The listing builds one solid part. Answer for the finished solid, in the listing's coordinates (mm). A direction names the side the tool comes from. Coordinates: 2 decimals unless noted, no trailing zeros. Order: outer loops, then holes, each group sorted by start corner. A loop starts at its lowest first (then second) coordinate and runs counter-clockwise, first axis right, second up. Notation, with made-up numbers: (65, 21.25) -> (120, 21.25) arc R34 cw to (120, 57.25) -> close; hole circle Ø11 at (84, 61). An arc over 180 degrees is marked (long way). Write each question's results on one line, items separated by ' | '. Start each with the question number.
(1) The part is cut by section C-C, the plane z = 6.25. Give the vertices of the cut face in (x, y), then the cut area to 3 significant figures.
(2) Straight lines are drawn through the part: L1, parallel to X at y = -30, z = 6.25; L2, parallel to Z at x = 46, y = 65.5; L3, parallel to Y at x = 44.5, z = 17. For each, find the intervals that lie inside material, in ascending order.
(3) The part is cut by section D-D, the plane y = 68. Give the vertices of the cut face in (x, z), then the cut area to 3 significant figures.
(4) The part is cut by section A-A, the plane z = 16.25. Give the vertices of the cut face in (x, y).
(5) A tool of negligible diameter and unlimited length cuts with its end or side. For faces 1 (the face through (19, -40.373, 6)), 2 (the face through (19, -41, 10)), 3 (the face through (58.3, 82.5, 13)), 4 (the face through (-15.649, 81, 13)), from which of +Z, -Z, +X, -X, +Y, -Y can it reach the whole face along a straight path? Write none if from no direction.
(6) The part is cut by section B-B, the plane x = 48. Give the vertices of the cut face in (y, z), then the cut area to 4 significant figures.
(7) Given pin 1 (8 mm diameter, centred on x = 3, z = 15, fed in from -Y); pin 2 (2.5 mm diameter, centred on x = 59, z = 16, fed in from -Y); pin 3 (8.5 mm diameter, centred on x = 6.5, y = 80.5, fed in from +Z), each flat-ended and moving along its own axis, determine where each tip first touches the part or whether it passes through.
```python
from build123d import *

# Parameters (mm, degrees)
IZIM1_W                     = 86
IZIM1_H                     = 136
IZIM1_W_2                   = 80
IZIM1_H_2                   = 130
Y_KSEKLIK_EKSTR_ZYON1_DEPTH = 10
IZIM1_2_W                   = 80
IZIM1_2_H                   = 130
Y_KSEKLIK_EKSTR_ZYON2_DEPTH = 3
Y_KSEKLIK_EKSTR_ZYON3_DEPTH = 86
KES_EKSTR_ZYON2_DEPTH       = 17
Y_KSEKLIK_EKSTR_ZYON4_REACH = 127.67


with BuildPart() as part:
    # Çizim1 → Yükseklik-Ekstrüzyon1 (new body)
    with BuildSketch(Plane.XY):
        with Locations((19.351242886, 24.627445339)):
            Rectangle(IZIM1_W, IZIM1_H)
        with Locations((19.351242886, 24.627445339)):
            Rectangle(IZIM1_W_2, IZIM1_H_2, mode=Mode.SUBTRACT)
    extrude(amount=Y_KSEKLIK_EKSTR_ZYON1_DEPTH)

    # Çizim1<2> → Yükseklik-Ekstrüzyon2 (add)
    with BuildSketch(Plane.XY):
        with Locations((19.351242886, 24.627445339)):
            Rectangle(IZIM1_2_W, IZIM1_2_H)
    extrude(amount=Y_KSEKLIK_EKSTR_ZYON2_DEPTH)

    # Çizim2 → Yükseklik-Ekstrüzyon3 (add, through all)
    with BuildSketch(Plane.ZY.offset(23.648757114)):
        with BuildLine():
            Line((18, 92.627445339), (10, 92.627445339))
            Line((10, 92.627445339), (10, 87.627445339))
            Line((10, 87.627445339), (10, 77.627445339))
            Line((10, 77.627445339), (10, 72.627445339))
            Line((10, 72.627445339), (18, 72.627445339))
            Line((18, 72.627445339), (18, 75.627445339))
            Line((18, 75.627445339), (18, 77.627445339))
            ThreePointArc((18, 77.627445339), (13, 82.627445339), (18, 87.627445339))
            Line((18, 87.627445339), (18, 89.627445339))
            Line((18, 89.627445339), (18, 92.627445339))
        make_face()
    extrude(amount=-Y_KSEKLIK_EKSTR_ZYON3_DEPTH)

    # Çizim5 → Kes-Ekstrüzyon2 (cut)
    with BuildSketch(Plane.XZ.offset(-72.627445339)):
        Polygon((-15.648757114, 10), (-15.648757114, 3), (54.351242886, 3), (54.351242886, 10), (54.351242886, 18), (-15.648757114, 18), align=None)
    extrude(amount=-KES_EKSTR_ZYON2_DEPTH, mode=Mode.SUBTRACT)

    # Yükseklik-Ekstrüzyon4: up to this face of the body (flat: up to its plane)
    y_kseklik_ekstr_zyon4_end = Plane(part.part.faces().sort_by_distance((59.351242886, 24.627445339, 6.5))[0])
    # Çizim6 → Yükseklik-Ekstrüzyon4 (add, up to the picked face)
    with BuildSketch(Plane(origin=(-20.648757114, 0, 0), x_dir=(0, 0, -1), z_dir=(1, 0, 0)), mode=Mode.PRIVATE) as y_kseklik_ekstr_zyon4_sk1:
        Polygon((-10, 72.627445339), (0, 82.627445339), (0, 92.627445339), (-10, 92.627445339), align=None)
    y_kseklik_ekstr_zyon4_tool1 = split(extrude(y_kseklik_ekstr_zyon4_sk1.sketch, amount=Y_KSEKLIK_EKSTR_ZYON4_REACH, mode=Mode.PRIVATE), bisect_by=y_kseklik_ekstr_zyon4_end, keep=Keep.BOTH, mode=Mode.PRIVATE)
    add(y_kseklik_ekstr_zyon4_tool1.solids().sort_by(Axis((-20.648757, 84.849668, 5.555556), (1, 0, 0)))[0])


solid = part.part
```
Established:
1) outline: (-23.65, -43.37) -> (62.35, -43.37) -> (62.35, 92.63) -> (-23.65, 92.63) -> close; hole (-20.65, -40.37) -> (59.35, -40.37) -> (59.35, 76.38) -> (-20.65, 76.38) -> close | area: 2,360 mm^2
2) L1: x = -23.65 to -20.65, 59.35 to 62.35 | L2: z = 0 to 3 | L3: y = 89.63 to 92.63
3) outline: (-23.65, 0) -> (62.35, 0) -> (62.35, 10) -> (59.35, 10) -> (59.35, 3) -> (-20.65, 3) -> (-20.65, 10) -> (-23.65, 10) -> close | area: 300 mm^2
4) outline: (-23.65, 72.63) -> (-15.65, 72.63) -> (-15.65, 77.94) -> (-23.65, 77.94) -> close; (-23.65, 87.31) -> (-15.65, 87.31) -> (-15.65, 89.63) -> (54.35, 89.63) -> (54.35, 87.31) -> (62.35, 87.31) -> (62.35, 92.63) -> (-23.65, 92.63) -> close; (54.35, 72.63) -> (62.35, 72.63) -> (62.35, 77.94) -> (54.35, 77.94) -> close
5) face 1: +Z | face 2: +Z, +X, -X, -Y | face 3: +Z, +X, -X | face 4: +Z, -Y
6) outline: (-43.37, 0) -> (92.63, 0) -> (92.63, 18) -> (89.63, 18) -> (89.63, 10) -> (72.63, 10) -> (79.63, 3) -> (-40.37, 3) -> (-40.37, 10) -> (-43.37, 10) -> close | area: 568.5 mm^2
7) pin 1: stops at y = 89.63 | pin 2: stops at y = 72.63 | pin 3: stops at z = 10
